```python
from build123d import *

# Parameters (mm, degrees)
SKETCH_1_W                   = 40
SKETCH_1_H                   = 8
EXTRUDE_1_DEPTH              = 39
HOLE_WIZARD_M4_2_D           = 3.3
HOLE_WIZARD_M4_2_DEPTH       = 8.1
HOLE_WIZARD_M4_2_CSINK_D     = 4.05
HOLE_WIZARD_M4_2_CSINK_ANGLE = 90
HOLE_WIZARD_M4_2_TIP         = 0.991420021
HOLE_WIZARD_M4_4_D           = 3.3
HOLE_WIZARD_M4_4_DEPTH       = 8.1
HOLE_WIZARD_M4_4_CSINK_D     = 4.05
HOLE_WIZARD_M4_4_CSINK_ANGLE = 90
HOLE_WIZARD_M4_4_TIP         = 0.991420021
SKETCH_11_R                  = 12.5
CUT_EXTRUDE_1_DEPTH          = 39
HOLE_WIZARD_M4_5_D           = 3.3
HOLE_WIZARD_M4_5_CSINK_D     = 4.05
HOLE_WIZARD_M4_5_CSINK_ANGLE = 90
SKETCH_14_W                  = 8
SKETCH_14_H                  = 8
CUT_EXTRUDE_2_DEPTH          = 8
HOLE_WIZARD_M4_6_D           = 3.3
HOLE_WIZARD_M4_6_CSINK_D     = 4.05
HOLE_WIZARD_M4_6_CSINK_ANGLE = 90
FILLET_1_R                   = 1
FILLET_2_R                   = 1


with BuildPart() as part:
    # 草图1 → 凸台-拉伸1 (new body)
    with BuildSketch(Plane(origin=(0, 0, 0), x_dir=(1, 0, 0), z_dir=(0, 1, 0))):
        Rectangle(SKETCH_1_W, SKETCH_1_H)
    extrude(amount=EXTRUDE_1_DEPTH)

    # M4 螺纹孔2
    with Locations(Plane(origin=(0, 39, 0), x_dir=(1, 0, 0), z_dir=(0, 1, 0))):
        with Locations((-15, 0), (15, 0)):
            CounterSinkHole(HOLE_WIZARD_M4_2_D / 2, HOLE_WIZARD_M4_2_CSINK_D / 2, depth=HOLE_WIZARD_M4_2_DEPTH, counter_sink_angle=HOLE_WIZARD_M4_2_CSINK_ANGLE)
            with Locations((0, 0, -(HOLE_WIZARD_M4_2_DEPTH + HOLE_WIZARD_M4_2_TIP / 2))):  # 118° drill point
                Cone(0, HOLE_WIZARD_M4_2_D / 2, HOLE_WIZARD_M4_2_TIP, mode=Mode.SUBTRACT)

    # M4 螺纹孔4
    with Locations(Plane(origin=(0, 0, 0), x_dir=(-1, 0, 0), z_dir=(0, -1, 0))):
        with Locations((15, 0), (-15, 0)):
            CounterSinkHole(HOLE_WIZARD_M4_4_D / 2, HOLE_WIZARD_M4_4_CSINK_D / 2, depth=HOLE_WIZARD_M4_4_DEPTH, counter_sink_angle=HOLE_WIZARD_M4_4_CSINK_ANGLE)
            with Locations((0, 0, -(HOLE_WIZARD_M4_4_DEPTH + HOLE_WIZARD_M4_4_TIP / 2))):  # 118° drill point
                Cone(0, HOLE_WIZARD_M4_4_D / 2, HOLE_WIZARD_M4_4_TIP, mode=Mode.SUBTRACT)

    # 草图11 → 切除-拉伸1 (cut)
    with BuildSketch(Plane.XY.offset(4)):
        with Locations((0, 23.5)):
            Circle(SKETCH_11_R)
    extrude(amount=-CUT_EXTRUDE_1_DEPTH, mode=Mode.SUBTRACT)

    # M4 螺纹孔5 (through all)
    with Locations(Plane(origin=(0, 39, 0), x_dir=(1, 0, 0), z_dir=(0, 1, 0))):
        with Locations((0, 0)):
            CounterSinkHole(HOLE_WIZARD_M4_5_D / 2, HOLE_WIZARD_M4_5_CSINK_D / 2, counter_sink_angle=HOLE_WIZARD_M4_5_CSINK_ANGLE)

    # 草图14 → 切除-拉伸2 (cut)
    with BuildSketch(Plane.XZ):
        Rectangle(SKETCH_14_W, SKETCH_14_H)
    extrude(amount=-CUT_EXTRUDE_2_DEPTH, mode=Mode.SUBTRACT)

    # M4 螺纹孔6 (through all)
    with Locations(Plane(origin=(20, 0, 0), x_dir=(0, 0, -1), z_dir=(1, 0, 0))):
        with Locations((0, 23.5)):
            CounterSinkHole(HOLE_WIZARD_M4_6_D / 2, HOLE_WIZARD_M4_6_CSINK_D / 2, counter_sink_angle=HOLE_WIZARD_M4_6_CSINK_ANGLE)

    # 圆角1
    fillet_1_edges = [part.edges().sort_by_distance(p)[0] for p in [
        (4, 8, 0),
        (-4, 8, 0),
    ]]
    fillet(fillet_1_edges, radius=FILLET_1_R)

    # 圆角2
    fillet_2_edges = [part.edges().sort_by_distance(p)[0] for p in [
        (20, 19.5, 4),
        (-20, 19.5, 4),
        (-20, 19.5, -4),
        (20, 19.5, -4),
    ]]
    fillet(fillet_2_edges, radius=FILLET_2_R)


solid = part.part
```
Geometry: final body of the model. Coordinates: model frame, mm. A direction names the side the tool comes from. Round coordinates to 2 decimals unless told otherwise and drop trailing zeros. Write each loop counter-clockwise with the first axis right and the second up, starting at its lowest first coordinate (ties: lowest second). Pieces come first, ordered by that corner, then holes. Notation, with made-up numbers: (35.5, 6) -> (57.5, 6) arc R31 ccw to (57.5, 40) -> close; hole circle Ø7 at (-32, 31). An arc over 180 degrees is marked (long way). Return JSON: item names as keys, results as strings.
Q1. Section B-B on z = -2.5. Return the cut outline in (x, y), and give its area (3 significant figures).
From the geometry:
{"outline": "(-20, 0) -> (-4, 0) -> (-4, 7) arc R1 cw to (-3, 8) -> (3, 8) arc R1 cw to (4, 7) -> (4, 0) -> (20, 0) -> (20, 39) -> (-20, 39) -> close; hole circle Ø25 at (0, 23.5)", "area": "1,010 mm2"}
Q2. First-contact query: pin 1 Ø2 at (x, z) = (0, 0) entering from +Y; pin 2 Ø2 at (x, z) = (-15, 0) entering from +Y; pin 3 Ø2 at (x, z) = (15, 0) entering from -Y; pin 4 Ø1.8 at (x, z) = (-1, -1.5) entering from -Y. Flat tips, straight axial feed; report the tip coordinate or a pass-through.
From the geometry:
{"pin 1": "through", "pin 2": "y = 30.51", "pin 3": "y = 8.49", "pin 4": "y = 8"}
Q3. Section A-A on y = 4. Return the cut outline in (x, z).
From the geometry:
{"outline": "(-20, -3) arc R1 ccw to (-19, -4) -> (-4, -4) -> (-4, 4) -> (-19, 4) arc R1 ccw to (-20, 3) -> close; (4, -4) -> (19, -4) arc R1 ccw to (20, -3) -> (20, 3) arc R1 ccw to (19, 4) -> (4, 4) -> close; hole circle Ø3.3 at (-15, 0); hole circle Ø3.3 at (15, 0)"}
Q4. Mould query, pull axis X, two halves, no side actions, for faces 1 (the cylindrical face through (1.216, 37.237, -1.115)), 2 (the cylindrical face through (19.699, 19.773, 3.715)), 3 (the flat face through (-20, 19, 0)). Classes: +X half, -X half, draft (parallel to the pull), parting line (faces both ways), or undercut.
From the geometry:
{"face 1": "undercut", "face 2": "+X half", "face 3": "-X half"}
Q5. Section C-C on y = 18.5. Return the cut outline in (x, z), and give its area (3 significant figures).
From the geometry:
{"outline": "(-20, -3) arc R1 ccw to (-19, -4) -> (-11.46, -4) -> (-11.46, 4) -> (-19, 4) arc R1 ccw to (-20, 3) -> close; (11.46, -4) -> (19, -4) arc R1 ccw to (20, -3) -> (20, 3) arc R1 ccw to (19, 4) -> (11.46, 4) -> close", "area": "136 mm2"}
Q6. Section D-D on x = -10.5. Return the cut outline in (y, z).
From the geometry:
{"outline": "(0, -4) -> (16.72, -4) -> (16.72, 4) -> (0, 4) -> close; (30.28, -4) -> (39, -4) -> (39, 4) -> (30.28, 4) -> close"}
Q7. Set-up query: faces 4 (the cylindrical face through (19.699, 19.773, -3.715)), 5 (the cylindrical face through (-13.476, 4.292, 0.632)), 6 (the cylindrical face through (-3.699, 7.715, 0.056)). Return all of +Z, -Z, +X, -X, +Y, -Y with unobstructed straight access to the full face (end or side cutting, diameter ignored); none if empty.
From the geometry:
{"face 4": "-Z, +X, +Y, -Y", "face 5": "-Y", "face 6": "+Z, -Z, -Y"}
Q8. Ray query, line 1 (Z direction, x = -15.25, y = 23.5); line 2 (X direction, y = 31, z = -1); line 3 (X direction, y = 36, z = 1.25). Return the intervals inside material, ascending.
From the geometry:
{"line 1": "-4 to -1.65, 1.65 to 4", "line 2": "-20 to -16.31, -13.69 to -10, 10 to 13.69, 16.31 to 20", "line 3": "-20 to -16.08, -13.92 to -1.08, 1.08 to 13.92, 16.08 to 20"}
